```python
from build123d import *

# Parameters (mm, degrees)
SZKIC1_R                    = 5
DODANIE_WYCI_GNI_CIE1_DEPTH = 1


with BuildPart() as part:
    # Szkic1 → Dodanie-wyciągnięcie1 (new body)
    with BuildSketch(Plane(origin=(0, 0, 0), x_dir=(1, 0, 0), z_dir=(0, 1, 0))):
        with BuildLine():
            Line((-12.5, 34.641016151), (12.5, 34.641016151))
            Line((12.5, 34.641016151), (45, 15.877132403))
            ThreePointArc((45, 15.877132403), (50.490381057, -4.613248654), (30, -10.103629711))
            Line((30, -10.103629711), (12.5, 0))
            Line((12.5, 0), (-12.5, 0))
            Line((-12.5, 0), (-30, -10.103629711))
            ThreePointArc((-30, -10.103629711), (-50.490381057, -4.613248654), (-45, 15.877132403))
            Line((-45, 15.877132403), (-12.5, 34.641016151))
        make_face()
        with Locations(Location((37.5, 2.886751346, 0), (0, 0, 270))):
            Circle(SZKIC1_R, mode=Mode.SUBTRACT)
        with Locations(Location((-37.5, 2.886751346, 0), (0, 0, 90))):
            Circle(SZKIC1_R, mode=Mode.SUBTRACT)
        with Locations(Location((0, 25.641016151, 0), (0, 0, 270))):
            Circle(SZKIC1_R, mode=Mode.SUBTRACT)
    extrude(amount=DODANIE_WYCI_GNI_CIE1_DEPTH)


solid = part.part
```
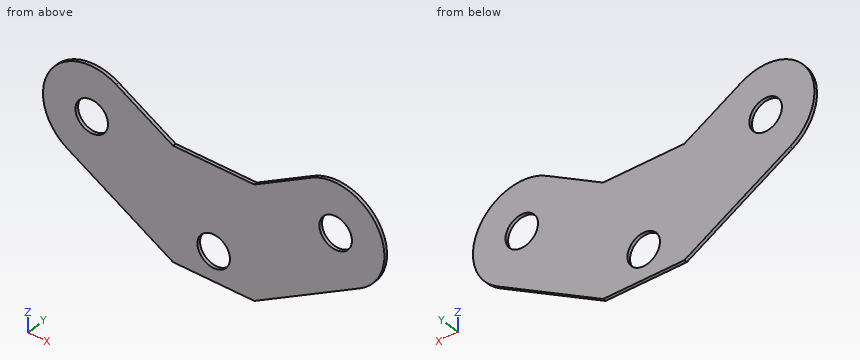
Source: CAD feature listing. Evaluate the final solid. Frame: model axes, mm. Give positions to 0.01 mm unless a question says otherwise; leave off trailing zeros. Order: outer loops, then holes, each group sorted by start corner. A loop starts at its lowest first (then second) coordinate and runs counter-clockwise, first axis right, second up.
(1) Section query C-C (y = 0.3). Return the cut outline in (x, z).
(2) Section query B-B (z = -4.5). Return the cut outline in (x, y).
(3) Material intervals for line 1 along X through (y, z) = (0.6, -2); line 2 along X through (y, z) = (0.8, 1.5); line 3 along X through (y, z) = (0.45, -28), sorted ascending.
(4) Section query A-A (x = 0). Return the cut outline in (y, z), plus the area to 3 significant figures.
(5) Section query D-D (z = -28). Return the cut outline in (x, y), plus the area to 3 significant figures.
Outcome:
1. outline: (-45, -15.88) - (-12.5, -34.64) - (12.5, -34.64) - (45, -15.88) arc R15 ccw to (30, 10.1) - (12.5, 0) - (-12.5, 0) - (-30, 10.1) arc R15 ccw to start; hole circle Ø10 at (-37.5, -2.89); hole circle Ø10 at (0, -25.64); hole circle Ø10 at (37.5, -2.89)
2. outline: (-52.41, 0) - (-42.23, 0) - (-42.23, 1) - (-52.41, 1) - close; (-32.77, 0) - (32.77, 0) - (32.77, 1) - (-32.77, 1) - close; (42.23, 0) - (52.41, 0) - (52.41, 1) - (42.23, 1) - close
3. line 1: x = -52.47 to -42.42, -32.58 to 32.58, 42.42 to 52.47
3. line 2: x = -51.84 to -39.9, -35.1 to -15.1, 15.1 to 35.1, 39.9 to 51.84
3. line 3: x = -24 to -4.41, 4.41 to 24
4. outline: (0, -34.64) - (1, -34.64) - (1, -30.64) - (0, -30.64) - close; (0, -20.64) - (1, -20.64) - (1, 0) - (0, 0) - close
4. area: 24.6 mm2
5. outline: (-24, 0) - (-4.41, 0) - (-4.41, 1) - (-24, 1) - close; (4.41, 0) - (24, 0) - (24, 1) - (4.41, 1) - close
5. area: 39.2 mm2
